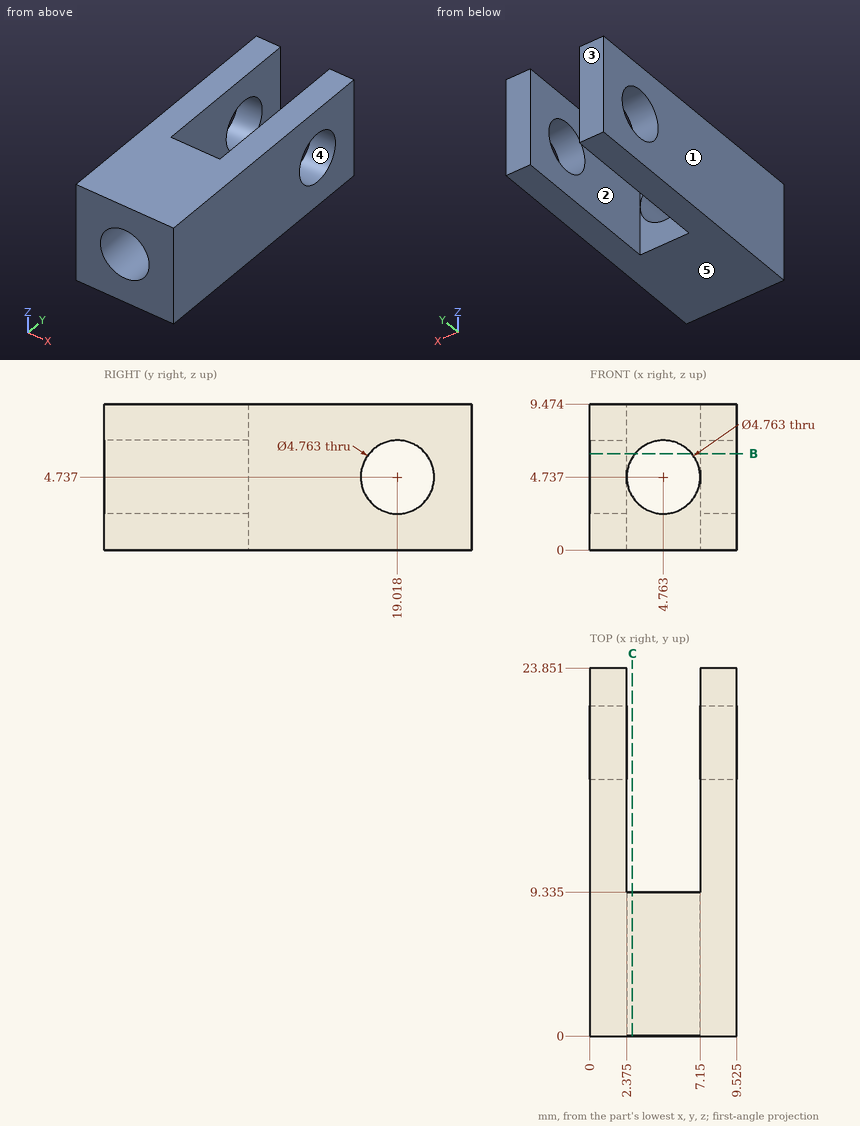
Input: dimensioned drawing with shaded views. Units: mm. Origin: part minimum x, y, z. A direction names the side the tool comes from. Round coordinates to 2 decimals unless told otherwise and drop trailing zeros. Order: outer loops, then holes, each group sorted by start corner. A loop starts at its lowest first (then second) coordinate and runs counter-clockwise, first axis right, second up. Notation, with made-up numbers: (6, 2.5) -> (31, 2.5) arc R15 cw to (31, 12.5) -> close; hole circle Ø5 at (86.5, 37.5). An arc over 180 degrees is marked (long way). One line per item, written item: value. Start each with the question number.
Q1. Access query for the marked faces 1 and 2. Directions: +Z, -Z, +X, -X, +Y, -Y. A direction counts if a zero-diameter tool reaches every point of the face in a straight line with its end or side. Return the directions, or none.
Q2. Section query B-B (z = 6.25). Give the number of separate pieces and of enclosed holes in the cut face, plus the area to 3 significant figures.
Q3. Section query C-C (x = 2.75). Return the cut outline in (y, z) (1 decimal).
Q4. Draft query along Z for the marked faces 3, 4 and 5. Return one class per face: pulls with the +Z half, pulls with the -Z half, needs draft (parallel to the pull), parting line crosses it, or undercut.
Q5. Pin query (flat end, axial travel): pin 1 (5 mm diameter, centred on y = 8, z = 4, fed in from -X); pin 2 (2.5 mm diameter, centred on x = 5.5, z = 3, fed in from +Y) (1 decimal). Return the tip coordinate at first contact, or that it passes through.
Q6. Material intervals for probe 1 along Z at (x, y) = (4.75, 1.75) (1 decimal); probe 2 along Y at (x, z) = (5, 7.25) (1 decimal); probe 3 along Z at (x, y) = (1.5, 21) (1 decimal), sorted ascending.
Findings below:
1. face 1: +Z, -Z, -X, +Y, -Y
1. face 2: +Z, -Z, +Y
2. separate pieces: 4
2. enclosed holes: 0
2. area: 106 mm²
3. outline: (0, 0) -> (9.3, 0) -> (9.3, 3.5) -> (0, 3.5) -> close; (0, 6) -> (9.3, 6) -> (9.3, 9.5) -> (0, 9.5) -> close
4. face 3: needs draft
4. face 4: undercut
4. face 5: pulls with the -Z half
5. pin 1: x = 0
5. pin 2: y = 9.3
6. probe 1: 0 to 2.4, 7.1 to 9.5
6. probe 2: 0 to 9.3
6. probe 3: 0 to 3.4, 6.1 to 9.5
